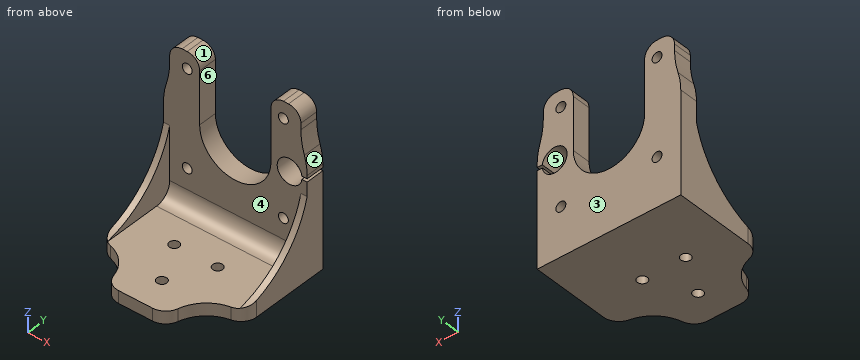
Autodesk Inventor part; units mm, degrees
ref_plane "YZ Plane" through (0, 0, 0) normal (1, 0, 0) x (0, 1, 0)
ref_plane "XZ Plane" through (0, 0, 0) normal (0, 1, 0) x (-1, 0, 0)
ref_plane "XY Plane" through (0, 0, 0) normal (0, 0, 1) x (1, 0, 0)
sketch "hole points" plane through (0, 0, 0) normal (0, 0, 1) x (1, 0, 0)
  line L0 (-7, 0) -> (7, 0) construction
  line L1 (0, 0) -> (0, -13) construction
  dimension "d0" = 14
  dimension "d1" = 13
sketch "Sketch3" plane through (0, 0, 0) normal (0, 0, 1) x (1, 0, 0)
  line L0 (-7, 0) -> (7, 0) construction
  line L1 (-7, 0) -> (7, 0) construction
  line L2 (-9, -2) -> (9, -2)
  line L3 (9, -2) -> (9, 2)
  line L4 (9, 2) -> (-9, 2)
  line L5 (-9, 2) -> (-9, -2)
  line L6 (-9, -2) -> (9, 2) construction
  line L7 (9, -2) -> (-9, 2) construction
  line L8 (0, 0) -> (0, -13) construction
  line L9 (-2, 2) -> (2, 2)
  line L10 (2, 2) -> (2, -15)
  line L11 (2, -15) -> (-2, -15)
  line L12 (-2, -15) -> (-2, 2)
  line L13 (17, -10) -> (-17, -10)
  line L14 (-17, -10) -> (-17, 10)
  line L15 (-17, 10) -> (17, 10)
  line L16 (17, 10) -> (17, -10)
  line L17 (10, -23) -> (10, 10)
  line L18 (10, 10) -> (-10, 10)
  line L19 (-10, 10) -> (-10, -23)
  line L20 (-10, -23) -> (10, -23)
  point P0 (0, -6.5)
  point P1 (0, 2)
  point P2 (0, -6.5)
  point P3 (0, 2)
  dimension "d31" = 18
  dimension "d32" = 4
  dimension "d33" = 4
  dimension "d34" = 17
  dimension "d35" = 8
  dimension "d36" = 8
extrude "back plate Extrusion2" add sketch "Sketch3" against normal blind 4
hole "Hole3" at (-7, 0, 0) at (7, 0, 0) at (0, -13, 0) direction (0, 0, -1) diameter 3.2 end through all
sketch "Sketch4" plane through (-17, 10, 0) normal (0, 1, 0) x (1, 0, 0)
  circle A0 centre (17.85, -27.15) radius 11
  circle A1 centre (2.35, -42.65) radius 1.5
  circle A2 centre (33.35, -11.65) radius 1.5
  circle A3 centre (33.35, -42.65) radius 1.5
  circle A4 centre (2.35, -11.65) radius 1.5
  line L0 (-3.3, -10) -> (0.7, -6)
  line L1 (-3.3, -44.3) -> (-3.3, -10)
  line L2 (0.7, -48.3) -> (-3.3, -44.3)
  line L3 (35, -48.3) -> (0.7, -48.3)
  line L4 (39, -44.3) -> (35, -48.3)
  line L5 (39, -10) -> (39, -44.3)
  line L6 (35, -6) -> (39, -10)
  line L7 (0.7, -6) -> (35, -6)
  line L8 (-3.3, 0) -> (39, 0)
  line L9 (39, 0) -> (39, 4)
  line L10 (39, 4) -> (-3.3, 4)
  line L11 (-3.3, 4) -> (-3.3, 0)
  line L12 (0, 4) -> (34, 4)
  point P0 (17, 0)
  point P1 (17.85, 4)
  point P2 (17, 4)
  point P3 (-3.3, 2)
  point P4 (39, 2)
  dimension "d44" = 4
extrude "Extrusion3" add sketch "Sketch4" along normal blind 10 contours L11 L10 L9 L8
sketch "Sketch5" plane through (0, 0, 0) normal (0, 0, 1) x (1, 0, 0)
  line L0 (-16.3, 14) -> (18, 14)
  line L1 (-20.3, 20) -> (22, 20)
  line L2 (22, 20) -> (22, 14)
  line L3 (22, 14) -> (-20.3, 14)
  line L4 (-20.3, 14) -> (-20.3, 20)
  point P0 (0, 0)
  dimension "d47" = 42.3
extrude "Extrusion4" add sketch "Sketch5" along normal blind 48
sketch "Sketch6" plane through (-17, 20, 0) normal (0, 1, 0) x (1, 0, 0)
  circle A0 centre (17.85, -27.15) radius 10.5
  circle A1 centre (17.85, -27.15) radius 11.5
  circle A2 centre (2.35, -42.65) radius 1.5 construction
  circle A3 centre (33.35, -42.65) radius 1.5 construction
  circle A4 centre (33.35, -11.65) radius 1.5 construction
  circle A5 centre (2.35, -11.65) radius 1.5 construction
  line L0 (6.35, -27.15) -> (6.35, -48)
  line L1 (39, -48) -> (-3.3, -48)
  line L2 (29.35, -27.15) -> (29.35, -48)
  line L3 (29.35, -48) -> (6.35, -48)
  point P0 (17, 0)
  dimension "d50" = 1
extrude "Extrusion5" cut sketch "Sketch6" against normal through all contours A0 | A1 | L2 L1 L0 A1
sketch "Sketch7" plane through (-17, 20, 0) normal (0, 1, 0) x (1, 0, 0)
  circle A0 centre (2.35, -42.65) radius 1.5
  circle A1 centre (33.35, -42.65) radius 1.5
  circle A2 centre (33.35, -11.65) radius 1.5
  circle A3 centre (2.35, -11.65) radius 1.5
  point P0 (17, 0)
hole "Hole4" at (-14.65, 20, 11.65) at (16.35, 20, 11.65) at (16.35, 20, 42.65) at (-14.65, 20, 42.65) direction (0, -1, 0) diameter 3.2 end through all
sketch "Sketch8" plane through (22, 10, 0) normal (1, 0, 0) x (0, 0, -1)
  line L0 (-24.65, 27.5) -> (-29.65, 27.5)
  line L1 (-22.15, 4) -> (-32.15, 4)
  line L2 (-32.15, 4) -> (-32.15, 10)
  line L3 (-32.15, 10) -> (-22.15, 10)
  line L4 (-22.15, 10) -> (-22.15, 4)
  point P0 (0, -10)
  point P1 (-27.15, 10)
  point P2 (-27.15, 27.5)
  point P3 (-27.15, 10)
  dimension "d62" = 10
  dimension "d63" = 6
extrude "Extrusion6" add sketch "Sketch8" along normal blind 2
sketch "Sketch9" plane through (-17, 20, 0) normal (0, 1, 0) x (1, 0, 0)
  circle A0 centre (17.85, -27.15) radius 2.5 construction
  line L0 (17.85, -27.15) -> (35.35, -27.15) construction
  point P0 (17, 0)
  dimension "d66" = 17.5
hole "Hole5" at (18.35, 20, 27.15) direction (0, -1, 0) diameter 8 end through all
sketch "Sketch10" plane through (24, 10, 0) normal (1, 0, 0) x (0, 0, -1)
  line L0 (-32.15, 4) -> (-22.15, 4)
  line L1 (-22.15, 4) -> (-22.15, 10)
  line L2 (-22.15, 10) -> (-32.15, 10)
  line L3 (-32.15, 10) -> (-32.15, 4)
  line L4 (-27.65, 10) -> (-26.65, 10)
  line L5 (-26.65, 10) -> (-26.65, 4)
  line L6 (-26.65, 4) -> (-27.65, 4)
  line L7 (-27.65, 4) -> (-27.65, 10)
  line L8 (-22.15, 10) -> (-32.15, 10)
  point P0 (0, -10)
  point P1 (-27.15, 10)
  point P2 (-27.15, 10)
  point P3 (-27.15, 10)
  dimension "d74" = 1
  dimension "d75" = 6
extrude "Extrusion7" cut sketch "Sketch10" against normal blind 5 contours L7 L2 L5 L0
sketch "Sketch11" plane through (-17, -10, -4) normal (-1, 0, 0) x (0, 0, 1)
  line L0 (4, 0) -> (4, 20)
  line L1 (4, 20) -> (0, 20)
  line L2 (0, 0) -> (0, 20)
  line L3 (4, 0) -> (0, 0)
  point P0 (4, 10)
extrude "Extrusion8" add sketch "Sketch11" along normal blind 3.3
sketch "Sketch12" plane through (17, -10, 0) normal (1, 0, 0) x (0, 0, -1)
  line L0 (0, 20) -> (0, 0)
  line L1 (0, 0) -> (4, 0)
  line L2 (4, 20) -> (4, 0)
  line L3 (0, 20) -> (4, 20)
  point P0 (0, 10)
extrude "Extrusion9" add sketch "Sketch12" along normal blind 5
fillet "Fillet3" radius 4 4 edges at (22, 17, 48) (12.35, 17, 48) (-10.65, 17, 48) (-20.3, 17, 48)
fillet "Fillet6" radius 5 1 edges at (0.85, 14, 0)
sketch "Sketch15" plane through (22, -10, -4) normal (1, 0, 0) x (0, 0, -1)
  line L0 (-26.15, 30) -> (-26.15, 24)
  line L1 (-9, 24) -> (-26.15, 24)
  arc A0 (-4, 19) -> (-9, 24) centre (-9, 19) ccw
  line L2 (-4, 0) -> (-4, 19)
  line L3 (-4, 0) -> (0, 0)
  line L4 (0, 0) -> (0, 30)
  line L5 (0, 30) -> (-26.15, 30)
  arc A1 (-4, 0) -> (-26.15, 24) centre (-33.5688, -5.0682) ccw
  line L6 (-26.15, 24) -> (-26.15, 30)
  line L7 (-26.15, 30) -> (0, 30)
  line L8 (0, 30) -> (-26.15, 30)
  line L9 (0, 30) -> (0, 0)
  line L10 (0, 0) -> (0, 30)
  line L11 (0, 0) -> (-4, 0)
  point P0 (-4, 10)
  dimension "d97" = 30
extrude "Extrusion12" add sketch "Sketch15" along normal blind 2
sketch "Sketch16" plane through (-20.3, -10, -4) normal (-1, 0, 0) x (0, 0, 1)
  line L0 (30.65, 30) -> (30.65, 24)
  line L1 (30.65, 24) -> (26.15, 24)
  arc A0 (26.15, 24) -> (4, 0) centre (33.5688, -5.0682) ccw
  line L2 (4, 0) -> (0, 0)
  line L3 (0, 0) -> (0, 30)
  line L4 (0, 30) -> (30.65, 30)
  point P0 (4, 10)
extrude "Extrusion13" add sketch "Sketch16" along normal blind 2
fillet "Fillet10" radius 12 2 edges at (-10, -10, -2) (10, -10, -2)
fillet "Fillet11" radius 5 4 edges at (-22.3, -10, -2) (-10, -23, -2) (10, -23, -2) (24, -10, -2)
sketch "Sketch17" plane through (-20.3, 14, 26.65) normal (0, 0, 1) x (1, 0, 0)
  line L0 (0, 6) -> (0, 0)
  line L1 (0, 6) -> (-2, 6)
  line L2 (-2, 0) -> (-2, 6)
  line L3 (0, 0) -> (-2, 0)
  point P0 (20.3, -14)
extrude "Extrusion14" add sketch "Sketch17" along normal blind 5.5
fillet "Fillet14" radius 25 2 edges at (-20.3, 17, 32.15) (22, 17, 32.15)
fillet "Fillet15" radius 20 2 edges at (-22.3, 17, 32.15) (24, 17, 32.15)
properties part number "bottom-right bracket" material "ABS Plastic"
Verification items for the finished model (mm, model axes). Face numbers are marked on the shaded views. A direction names the side the tool comes from. Round coordinates to 2 decimals unless told otherwise and drop trailing zeros. Loops run counter-clockwise (first coordinate to the right, second up) from the corner with the lowest first, then second, coordinate; pieces in that order, holes last. Notation, with made-up numbers: (2, 51) - (12, 51) arc R20 ccw to (12, 68) - close; hole circle Ø8 at (-28.5, -21.75). An arc over 180 degrees is marked (long way). Answer in a Markdown table with one row per item. Add a question column.
Q1. Material ranges on line 1 (X direction, y = 16.8, z = 42.65); line 2 (X direction, y = 0, z = -2); line 3 (Z direction, x = -14.65, y = 17.45), recorded low to high.
Q2. Gauge pin test, flat ends, axial feed: pin 1 (1.6 mm diameter, centred on y = 18, z = 43.5, fed in from +X); pin 2 (1.5 mm diameter, centred on x = 19.5, y = 7, fed in from +Z); pin 3 (2.5 mm diameter, centred on x = 7, y = 0, fed in from -Z); pin 4 (5 mm diameter, centred on x = 18, z = 41, fed in from -Y). Record the tip position at first contact, or that the pin passes through.
Q3. Tool access check on the marked faces 4, 5 and 6. Record the directions out of +Z, -Z, +X, -X, +Y, -Y that give a thin tool (end or side, any length) a straight path to the whole face; none if there is none.
Q4. Section check C-C on z = 11.65. Enter the section's corners in (x, y), plus the area to 3 significant figures.
Q5. Section check A-A on y = 16. Enter the section's corners in (x, z).
Q6. Section check D-D on x = -7. Enter the section's corners in (y, z), plus the area to 3 significant figures.
Q7. Release check for a two-part mould opening along X. For the marked faces 1, 2 and 3 record: pulls with the +X half, pulls with the -X half, needs draft (parallel to the pull), parting line crosses it, or undercut.
Q8. Section check B-B on y = 0. Enter the section's corners in (x, z).
Found:
| question | item | result |
|---|---|---|
| 1 | line 1 | x = -20.3 to -16.25, -13.05 to -10.65, 12.35 to 14.75, 17.95 to 22 |
| 1 | line 2 | x = -22.3 to -8.6, -5.4 to 5.4, 8.6 to 24 |
| 1 | line 3 | z = -4 to 10.05, 13.25 to 41.05, 44.25 to 48 |
| 2 | pin 1 | stops at x = 22 |
| 2 | pin 2 | stops at z = 0 |
| 2 | pin 3 | passes through |
| 2 | pin 4 | stops at y = 14 |
| 3 | face 4 | +Z, -Y |
| 3 | face 5 | +Y, -Y |
| 3 | face 6 | +Z, +Y, -Y |
| 4 | outline | (-22.3, 8.99) - (-20.3, 8.99) - (-20.3, 14) - (-16.25, 14) - (-16.25, 20) - (-22.3, 20) - close; (-13.05, 14) - (14.75, 14) - (14.75, 20) - (-13.05, 20) - close; (17.95, 14) - (22, 14) - (22, 8.99) - (24, 8.99) - (24, 20) - (17.95, 20) - close |
| 4 | area | 259 mm² |
| 5 | outline | (-22.3, -4) - (24, -4) - (24, 26.65) - (22.32, 26.65) arc R4 cw (long way) to (22.32, 27.65) - (24, 27.65) - (24, 28.68) arc R20 ccw to (23.11, 34.58) arc R25 cw to (22, 41.95) - (22, 44) arc R4 ccw to (18, 48) - (16.35, 48) arc R4 ccw to (12.35, 44) - (12.35, 27.15) arc R11.5 cw to (-10.65, 27.15) - (-10.65, 44) arc R4 ccw to (-14.65, 48) - (-16.3, 48) arc R4 ccw to (-20.3, 44) - (-20.3, 41.95) arc R25 cw to (-21.41, 34.58) arc R20 ccw to (-22.3, 28.68) - close; hole circle Ø3.2 at (-14.65, 11.65); hole circle Ø3.2 at (-14.65, 42.65); hole circle Ø3.2 at (16.35, 11.65); hole circle Ø3.2 at (16.35, 42.65) |
| 6 | outline | (-22.76, -4) - (-1.6, -4) - (-1.6, 0) - (-22.76, 0) - close; (1.6, -4) - (20, -4) - (20, 18.75) - (14, 18.75) - (14, 5) arc R5 cw to (9, 0) - (1.6, 0) - close |
| 6 | area | 276 mm² |
| 7 | face 1 | undercut |
| 7 | face 2 | pulls with the +X half |
| 7 | face 3 | needs draft |
| 8 | outline | (-22.3, -4) - (-8.6, -4) - (-8.6, 0) - (-20.3, 0) - (-20.3, 3.63) - (-22.3, 3.63) - close; (-5.4, -4) - (5.4, -4) - (5.4, 0) - (-5.4, 0) - close; (8.6, -4) - (24, -4) - (24, 3.63) - (22, 3.63) - (22, 0) - (8.6, 0) - close |
